```python
from build123d import *

# Parameters (mm, degrees)
SKETCH1_R           = 42
SKETCH1_R_2         = 1.95
SKETCH1_R_3         = 3.55
SKETCH1_R_4         = 1.45
BOSS_EXTRUDE1_DEPTH = 8
CUT_EXTRUDE2_DEPTH  = 10
SKETCH4_W           = 3.8
SKETCH4_H           = 3.8
CUT_EXTRUDE3_DEPTH  = 35
SKETCH5_R           = 12
SKETCH5_R_2         = 1.45
BOSS_EXTRUDE2_DEPTH = 3


with BuildPart() as part:
    # Sketch1 → Boss-Extrude1 (new body)
    with BuildSketch(Plane(origin=(0, 0, 0), x_dir=(1, 0, 0), z_dir=(0, 1, 0))):
        Circle(SKETCH1_R)
        with Locations((0, 18)):
            Circle(SKETCH1_R_2, mode=Mode.SUBTRACT)
        with Locations((15.588457268, -9)):
            Circle(SKETCH1_R_2, mode=Mode.SUBTRACT)
        with Locations((-15.588457268, -9)):
            Circle(SKETCH1_R_2, mode=Mode.SUBTRACT)
        Circle(SKETCH1_R_3, mode=Mode.SUBTRACT)
        with Locations((7.794228634, 4.5)):
            Circle(SKETCH1_R_4, mode=Mode.SUBTRACT)
        with Locations((0, -9)):
            Circle(SKETCH1_R_4, mode=Mode.SUBTRACT)
        with Locations((-7.794228634, 4.5)):
            Circle(SKETCH1_R_4, mode=Mode.SUBTRACT)
    extrude(amount=BOSS_EXTRUDE1_DEPTH)

    # Sketch3 → Cut-Extrude2 (cut)
    with BuildSketch(Plane(origin=(0, 8, 0), x_dir=(1, 0, 0), z_dir=(0, 1, 0))):
        with BuildLine():
            Line((0.5, 7), (0.5, 0))
            ThreePointArc((0.5, 0), (0, -0.5), (-0.5, 0))
            Line((-0.5, 0), (-0.5, 7))
            ThreePointArc((-0.5, 7), (0, 7.5), (0.5, 7))
        make_face()
    extrude(amount=-CUT_EXTRUDE2_DEPTH, mode=Mode.SUBTRACT)

    # Sketch4 → Cut-Extrude3 (cut)
    with BuildSketch(Plane(origin=(0, 8, 0), x_dir=(1, 0, 0), z_dir=(0, 1, 0))):
        Polygon((1.905255888, -16.9), (5.196152423, -15), (3.296152423, -11.709103466), (0.005255888, -13.609103466), align=None)
        with Locations((-13.688457268, 4.9)):
            Rectangle(SKETCH4_W, SKETCH4_H)
        Polygon((13.68320138, 10.1), (10.392304845, 12), (8.492304845, 8.709103466), (11.78320138, 6.809103466), align=None)
    extrude(amount=-CUT_EXTRUDE3_DEPTH, mode=Mode.SUBTRACT)

    # Sketch5 → Boss-Extrude2 (add)
    with BuildSketch(Plane.XZ):
        Circle(SKETCH5_R)
        with Locations((0, 9)):
            Circle(SKETCH5_R_2, mode=Mode.SUBTRACT)
        with Locations((-7.794228634, -4.5)):
            Circle(SKETCH5_R_2, mode=Mode.SUBTRACT)
        with Locations((7.794228634, -4.5)):
            Circle(SKETCH5_R_2, mode=Mode.SUBTRACT)
        with BuildLine():
            Line((-0.5, -7), (-0.5, -3.514612354))
            ThreePointArc((-0.5, -3.514612354), (0, 3.55), (0.5, -3.514612354))
            Line((0.5, -3.514612354), (0.5, -7))
            ThreePointArc((0.5, -7), (0, -7.5), (-0.5, -7))
        make_face(mode=Mode.SUBTRACT)
    extrude(amount=BOSS_EXTRUDE2_DEPTH)


solid = part.part
```
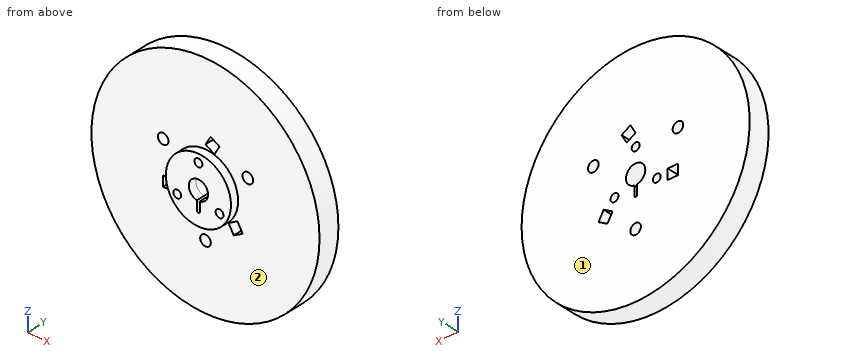
Verification items for the finished model (mm, model axes). Face numbers are marked on the shaded views. A direction names the side the tool comes from. Give positions to 0.01 mm unless a question says otherwise; leave off trailing zeros. Loops run counter-clockwise (first coordinate to the right, second up) from the corner with the lowest first, then second, coordinate; pieces in that order, holes last.
1. Set-up check for the marked faces 1 and 2: record each of +Z, -Z, +X, -X, +Y, -Y from which the full face is reachable in a straight line by a thin tool's end or side.
2. Section check C-C, the plane x = 16.5. Enter the section's corners in (y, z).
3. Go/stop test with flat-tipped pins: pin 1 Ø1.7 at (y, z) = (5, -5.5) entering from -X; pin 2 Ø1.1 at (x, y) = (-14, 6) entering from -Z; pin 3 Ø4 at (y, z) = (0.5, -20) entering from -X. Record where each tip stops, or that it passes through.
4. Section check B-B, the plane y = -2. Enter the section's corners in (x, z), then the cut area to 3 significant figures.
5. Section check A-A, the plane z = 0. Enter the section's corners in (x, y), then the cut area to 3 significant figures.
6. Section check D-D, the plane z = 9. Enter the section's corners in (x, y), then the cut area to 3 significant figures.
7. Thickness scan on line 1 (X direction, y = 1.75, z = 9); line 2 (Y direction, x = -0.5, z = 38); line 3 (Z direction, x = -8.5, y = 3.5). Record the ranges inside material, lowest first.
Geometry says:
1. face 1: +Z, -Z, +X, -X, +Y
1. face 2: -Y
2. outline: (0, -38.62) - (8, -38.62) - (8, 7.28) - (0, 7.28) - close; (0, 10.72) - (8, 10.72) - (8, 38.62) - (0, 38.62) - close
3. pin 1: stops at x = -41.74
3. pin 2: stops at z = -39.79
3. pin 3: stops at x = -37.95
4. outline: circle Ø24 at (0, 0); hole circle Ø2.9 at (-7.79, -4.5); hole circle Ø2.9 at (0, 9); hole (-0.5, -7) arc R0.5 ccw to (0.5, -7) - (0.5, -3.51) arc R3.55 ccw (long way) to (-0.5, -3.51) - close; hole circle Ø2.9 at (7.79, -4.5)
4. area: 389 mm2
5. outline: (-42, 0) - (-12, 0) - (-12, -3) - (-3.55, -3) - (-3.55, 8) - (-42, 8) - close; (3.55, -3) - (12, -3) - (12, 0) - (42, 0) - (42, 8) - (3.55, 8) - close
5. area: 666 mm2
6. outline: (-41.02, 0) - (-17.54, 0) - (-17.54, 8) - (-41.02, 8) - close; (-13.64, 0) - (-7.94, 0) - (-7.94, -3) - (-1.45, -3) - (-1.45, 8) - (-13.64, 8) - close; (1.45, -3) - (7.94, -3) - (7.94, 0) - (13.64, 0) - (13.64, 8) - (1.45, 8) - close; (17.54, 0) - (41.02, 0) - (41.02, 8) - (17.54, 8) - close
6. area: 610 mm2
7. line 1: x = -41.02 to -17.54, -13.64 to -1.45, 1.45 to 13.64, 17.54 to 41.02
7. line 2: y = 0 to 8
7. line 3: z = -41.13 to -5.77, -3.23 to 41.13
